Input: part model. Units: mm. Frame: model coordinates. A direction names the side the tool comes from. Round coordinates to 2 decimals unless told otherwise and drop trailing zeros. Loops run counter-clockwise (first coordinate to the right, second up) from the corner with the lowest first, then second, coordinate; pieces in that order, holes last. Notation, with made-up numbers: (34, 88) - (73, 88) arc R24 cw to (73, 98) - close; hole circle Ø9 at (84, -36.75). An arc over 180 degrees is marked (long way). Write each question's results on one line, items separated by ' | '.
from build123d import *

# Parameters (mm, degrees)
F0_W     = 6
F0_H     = 0.8
F0_H_2   = 0.4
F1_DEPTH = 1
F2_DEPTH = 5
F3_DEPTH = 2.4
F5_DEPTH = 1
F6_R     = 0.2


with BuildPart() as f1:
    # F0 (on Top) → F1 (new body)
    with BuildSketch(Plane.XY):
        with Locations((0, -0.6)):
            Rectangle(F0_W, F0_H)
        Rectangle(F0_W, F0_H_2)
        with Locations((0, 0.6)):
            Rectangle(F0_W, F0_H)
    extrude(amount=-F1_DEPTH)

    # F0 (on Top) → F2 (join)
    with BuildSketch(Plane.XY):
        with Locations((0, 0.6)):
            Rectangle(F0_W, F0_H)
    extrude(amount=F2_DEPTH)

    # F0 (on Top) → F3 (join)
    with BuildSketch(Plane.XY):
        with Locations((0, -0.6)):
            Rectangle(F0_W, F0_H)
    extrude(amount=F3_DEPTH)

    # F4 (on face) → F5 (cut)
    with BuildSketch(Plane.XZ.offset(1)):
        Polygon((-3, 2.4), (-3, 0.7), (0, 2.4), align=None)
        Polygon((3, 2.4), (0, 2.4), (3, 0.7), align=None)
    extrude(amount=-F5_DEPTH, mode=Mode.SUBTRACT)

    # F6
    f6_edges = [f1.edges().sort_by_distance(p)[0] for p in [
        (3, 0.6, 5),
        (-3, 0.6, 5),
        (3, 0, -1),
        (-3, 0, -1),
        (3, 1, 2),
        (-3, 1, 2),
        (3, -1, -0.15),
        (-3, -1, -0.15),
        (-1.5, -1, 1.55),
        (1.5, -1, 1.55),
        (0, 1, 5),
    ]]
    fillet(f6_edges, radius=F6_R)


solid = f1.part
1. Section query C-C, the plane z = 3.05. Output: boundary loops of the cut face in (x, y), plus the area to 3 significant figures.
Answer:
outline: (-3, 0.2) - (3, 0.2) - (3, 0.8) arc R0.2 ccw to (2.8, 1) - (-2.8, 1) arc R0.2 ccw to (-3, 0.8) - close | area: 4.78 mm^2
2. Set-up query: faces 4 (the flat face through (0, 1, 2)), 5 (the flat face through (1.48, -0.5, 1.56)), 6 (the flat face through (0, 0.2, 2)). Return all of +Z, -Z, +X, -X, +Y, -Y with unobstructed straight access to the full face (end or side cutting, diameter ignored); none if empty.
Answer:
face 4: +Z, -Z, +X, -X, +Y | face 5: +Z, +X, -Y | face 6: +Z, +X, -X
3. Line query: line 1 (Y direction, x = 0.25, z = 0.55); line 2 (Y direction, x = -1.75, z = 1.5); line 3 (Z direction, x = 0.5, y = 0.15). Output: solid intervals per line, ascending. Write a range as [from, to].
Answer:
line 1: [-1, -0.2], [0.2, 1] | line 2: [0.2, 1] | line 3: [-1, 0]
4. Section query B-B, the plane y = -0.45. Output: boundary loops of the cut face in (x, z).
Answer:
outline: (-3, -0.8) arc R0.2 ccw to (-2.8, -1) - (2.8, -1) arc R0.2 ccw to (3, -0.8) - (3, 0.7) - (0, 2.4) - (-3, 0.7) - close
5. Mould query, pull axis Y, two halves, no side actions, for faces 1 (the flat face through (0, -1, 0)), 2 (the flat face through (0, -0.2, 1)), 3 (the flat face through (-1.52, -0.5, 1.54)). Classes: pulls with the +Y half, pulls with the -Y half, needs draft (parallel to the pull), parting line crosses it, or undercut.
Answer:
face 1: pulls with the -Y half | face 2: undercut | face 3: needs draft
6. Section query D-D, the plane y = 0. Output: boundary loops of the cut face in (x, z), plus the area to 3 significant figures.
Answer:
outline: (-3, -0.8) arc R0.2 ccw to (-2.8, -1) - (2.8, -1) arc R0.2 ccw to (3, -0.8) - (3, 0) - (-3, 0) - close | area: 5.98 mm^2
7. Section query A-A, the plane z = 0.3. Output: boundary loops of the cut face in (x, y).
Answer:
outline: (-3, -0.8) arc R0.2 ccw to (-2.8, -1) - (2.8, -1) arc R0.2 ccw to (3, -0.8) - (3, -0.2) - (-3, -0.2) - close; (-3, 0.2) - (3, 0.2) - (3, 0.8) arc R0.2 ccw to (2.8, 1) - (-2.8, 1) arc R0.2 ccw to (-3, 0.8) - close
